Geometry check sheet. Reference: the model listing, model coordinates, mm. A direction names the side the tool comes from. Round coordinates to 2 decimals unless told otherwise and drop trailing zeros. Loops run counter-clockwise (first coordinate to the right, second up) from the corner with the lowest first, then second, coordinate; pieces in that order, holes last. Notation, with made-up numbers: (50.25, 52) -> (75.25, 52) arc R21 cw to (75.25, 79) -> close; hole circle Ø3 at (-32.5, -30). An arc over 180 degrees is marked (long way). Use a Markdown table: item, result. Add a question column.
Q1. Sectioned sample at A-A, the plane z = -48.5. Enter the section's corners in (x, y).
Q2. Release check for a two-part mould opening along Z. For faces 4 (the face through (16.25, 1.52, -310.3)), 5 (the face through (203.75, 1.52, -9.7)), 6 (the face through (41.01, 1.52, -283.15)) record: released by +Z, released by -Z, zero draft, split by the parting line, or undercut.
Q3. Set-up check for faces 1 (the face through (9.67, 1.52, -18.96)), 2 (the face through (47.85, 1.52, -207.99)), 3 (the face through (16.065, 1.521, -9.482)): record each of +Z, -Z, +X, -X, +Y, -Y from which the full face is reachable in a straight line by a thin tool's end or side.
Q4. Material ranges on L1, parallel to X at y = 2.05, z = -119.5; L2, parallel to X at y = 2.35, z = -44; L3, parallel to X at y = 1.6, z = -104.5, recorded low to high.
Q5. Sectioned sample at C-C, the plane y = 2.05. Give the number of separate pieces and of enclosed holes in the cut face, then the cut area to 3 significant figures.
Q6. Sectioned sample at B-B, the plane x = 144.5. Enter the section's corners in (y, z), then the cut area to 3 significant figures.
Q7. Gauge pin test, flat ends, axial feed: P1, Ø1.5, axis at y = 2, z = -136.5, coming from the -X side; P2, Ø1.5, axis at x = 23, y = 1.5, coming from the -Z side; P3, Ø0.9, axis at y = 2, z = -189, coming from the +X side. Record the tip position at first contact, or that the pin passes through.
```python
from build123d import *

# Parameters (mm, degrees)
CROQUIS1_W              = 220
CROQUIS1_H              = 320
CROQUIS1_R              = 1.7
CROQUIS1_R_2            = 1.6
SALIENTE_EXTRUIR1_DEPTH = 3
CROQUIS2_OUTSIDE_W      = 299.668
CROQUIS2_OUTSIDE_H      = 399.668
CORTAR_EXTRUIR1_DEPTH   = 3
REDONDEO1_R             = 5
CROQUIS3_W              = 20
CROQUIS3_H              = 45
CORTAR_EXTRUIR2_DEPTH   = 3
CROQUIS4_W              = 15
CROQUIS4_H              = 60
CORTAR_EXTRUIR3_DEPTH   = 3
REDONDEO2_R             = 5


with BuildPart() as part:
    # Croquis1 → Saliente-Extruir1 (new body)
    with BuildSketch(Plane(origin=(0, 0, 0), x_dir=(1, 0, 0), z_dir=(0, 1, 0))):
        with Locations((110, 160)):
            Rectangle(CROQUIS1_W, CROQUIS1_H)
        with Locations(Location((185, 167.5, 0), (0, 0, 270))):
            Circle(CROQUIS1_R, mode=Mode.SUBTRACT)
        with Locations(Location((205, 167.5, 0), (0, 0, 270))):
            Circle(CROQUIS1_R, mode=Mode.SUBTRACT)
        with Locations(Location((185, 152.5, 0), (0, 0, 90))):
            Circle(CROQUIS1_R, mode=Mode.SUBTRACT)
        with Locations(Location((205, 152.5, 0), (0, 0, 90))):
            Circle(CROQUIS1_R, mode=Mode.SUBTRACT)
        with Locations(Location((35, 215.5, 0), (0, 0, 270))):
            Circle(CROQUIS1_R, mode=Mode.SUBTRACT)
        with Locations(Location((35, 200.5, 0), (0, 0, 270))):
            Circle(CROQUIS1_R, mode=Mode.SUBTRACT)
        with Locations(Location((35, 119.5, 0), (0, 0, 90))):
            Circle(CROQUIS1_R, mode=Mode.SUBTRACT)
        with Locations(Location((35, 104.5, 0), (0, 0, 90))):
            Circle(CROQUIS1_R, mode=Mode.SUBTRACT)
        with Locations(Location((5.5, 314.5, 0), (0, 0, 270))):
            Circle(CROQUIS1_R_2, mode=Mode.SUBTRACT)
        with Locations(Location((214.5, 314.5, 0), (0, 0, 90))):
            Circle(CROQUIS1_R_2, mode=Mode.SUBTRACT)
        with Locations(Location((214.5, 5.5, 0), (0, 0, 270))):
            Circle(CROQUIS1_R_2, mode=Mode.SUBTRACT)
        with Locations(Location((5.5, 5.5, 0), (0, 0, 90))):
            Circle(CROQUIS1_R_2, mode=Mode.SUBTRACT)
        with Locations(Location((15, 200.5, 0), (0, 0, 90))):
            Circle(CROQUIS1_R, mode=Mode.SUBTRACT)
        with Locations(Location((15, 215.5, 0), (0, 0, 90))):
            Circle(CROQUIS1_R, mode=Mode.SUBTRACT)
        with Locations(Location((15, 104.5, 0), (0, 0, 270))):
            Circle(CROQUIS1_R, mode=Mode.SUBTRACT)
        with Locations(Location((15, 119.5, 0), (0, 0, 270))):
            Circle(CROQUIS1_R, mode=Mode.SUBTRACT)
        with Locations(Location((110, 180, 0), (0, 0, 270))):
            Circle(CROQUIS1_R_2, mode=Mode.SUBTRACT)
        with Locations(Location((110, 140, 0), (0, 0, 90))):
            Circle(CROQUIS1_R_2, mode=Mode.SUBTRACT)
        with Locations(Location((5.5, 160, 0), (0, 0, 270))):
            Circle(CROQUIS1_R_2, mode=Mode.SUBTRACT)
        with Locations(Location((214.5, 160, 0), (0, 0, 90))):
            Circle(CROQUIS1_R_2, mode=Mode.SUBTRACT)
    extrude(amount=SALIENTE_EXTRUIR1_DEPTH)

    # Croquis2 outside → Cortar-Extruir1 (cut)
    # profile 1 of 9: a face of its own
    with BuildSketch(Plane(origin=(0, 3, 0), x_dir=(1, 0, 0), z_dir=(0, 1, 0))):
        with Locations((110, 160)):
            Rectangle(CROQUIS2_OUTSIDE_W, CROQUIS2_OUTSIDE_H)
        with BuildLine():
            Line((9, 148.77502784), (9, 94.5))
            Line((9, 94.5), (19, 94.5))
            Line((19, 94.5), (19, 30))
            Line((19, 30), (1.298802547, 9.049639413))
            ThreePointArc((1.298802547, 9.049639413), (1.950360587, 1.298802547), (9.701197453, 1.950360587))
            Line((9.701197453, 1.950360587), (24.106631311, 19))
            Line((24.106631311, 19), (195.893368689, 19))
            Line((195.893368689, 19), (210.298802547, 1.950360587))
            ThreePointArc((210.298802547, 1.950360587), (218.049639413, 1.298802547), (218.701197453, 9.049639413))
            Line((218.701197453, 9.049639413), (201, 30))
            Line((201, 30), (201, 94.5))
            Line((201, 94.5), (211, 94.5))
            Line((211, 94.5), (211, 148.77502784))
            ThreePointArc((211, 148.77502784), (212.318863014, 152.528287293), (215.695652174, 154.631535054))
            ThreePointArc((215.695652174, 154.631535054), (220, 160), (215.695652174, 165.368464946))
            ThreePointArc((215.695652174, 165.368464946), (212.318863014, 167.471712707), (211, 171.22497216))
            Line((211, 171.22497216), (211, 225.5))
            Line((211, 225.5), (201, 225.5))
            Line((201, 225.5), (201, 290))
            Line((201, 290), (218.701197453, 310.950360587))
            ThreePointArc((218.701197453, 310.950360587), (218.049639413, 318.701197453), (210.298802547, 318.049639413))
            Line((210.298802547, 318.049639413), (195.893368689, 301))
            Line((195.893368689, 301), (24.106631311, 301))
            Line((24.106631311, 301), (9.701197453, 318.049639413))
            ThreePointArc((9.701197453, 318.049639413), (1.950360587, 318.701197453), (1.298802547, 310.950360587))
            Line((1.298802547, 310.950360587), (19, 290))
            Line((19, 290), (19, 225.5))
            Line((19, 225.5), (9, 225.5))
            Line((9, 225.5), (9, 171.22497216))
            ThreePointArc((9, 171.22497216), (7.681136986, 167.471712707), (4.304347826, 165.368464946))
            ThreePointArc((4.304347826, 165.368464946), (0, 160), (4.304347826, 154.631535054))
            ThreePointArc((4.304347826, 154.631535054), (7.681136986, 152.528287293), (9, 148.77502784))
        make_face(mode=Mode.SUBTRACT)
    # profile 2 of 9: a face of its own
    with BuildSketch(Plane(origin=(0, 3, 0), x_dir=(1, 0, 0), z_dir=(0, 1, 0))):
        with BuildLine():
            Line((182, 276), (182, 236))
            ThreePointArc((182, 236), (179.071067812, 228.928932188), (172, 226))
            Line((172, 226), (118, 226))
            ThreePointArc((118, 226), (116.585786438, 226.585786438), (116, 228))
            Line((116, 228), (116, 284))
            ThreePointArc((116, 284), (116.585786438, 285.414213562), (118, 286))
            Line((118, 286), (172, 286))
            ThreePointArc((172, 286), (179.071067812, 283.071067812), (182, 276))
        make_face()
    # profile 3 of 9: a face of its own
    with BuildSketch(Plane(origin=(0, 3, 0), x_dir=(1, 0, 0), z_dir=(0, 1, 0))):
        with BuildLine():
            Line((102, 286), (48, 286))
            ThreePointArc((48, 286), (40.928932188, 283.071067812), (38, 276))
            Line((38, 276), (38, 236))
            ThreePointArc((38, 236), (40.928932188, 228.928932188), (48, 226))
            Line((48, 226), (102, 226))
            ThreePointArc((102, 226), (103.414213562, 226.585786438), (104, 228))
            Line((104, 228), (104, 284))
            ThreePointArc((104, 284), (103.414213562, 285.414213562), (102, 286))
        make_face()
    # profile 4 of 9: a face of its own
    with BuildSketch(Plane(origin=(0, 3, 0), x_dir=(1, 0, 0), z_dir=(0, 1, 0))):
        with BuildLine():
            Line((102, 94), (48, 94))
            ThreePointArc((48, 94), (40.928932188, 91.071067812), (38, 84))
            Line((38, 84), (38, 44))
            ThreePointArc((38, 44), (40.928932188, 36.928932188), (48, 34))
            Line((48, 34), (102, 34))
            ThreePointArc((102, 34), (103.414213562, 34.585786438), (104, 36))
            Line((104, 36), (104, 92))
            ThreePointArc((104, 92), (103.414213562, 93.414213562), (102, 94))
        make_face()
    # profile 5 of 9: a face of its own
    with BuildSketch(Plane(origin=(0, 3, 0), x_dir=(1, 0, 0), z_dir=(0, 1, 0))):
        with BuildLine():
            Line((116, 36), (116, 92))
            ThreePointArc((116, 92), (116.585786438, 93.414213562), (118, 94))
            Line((118, 94), (172, 94))
            ThreePointArc((172, 94), (179.071067812, 91.071067812), (182, 84))
            Line((182, 84), (182, 44))
            ThreePointArc((182, 44), (179.071067812, 36.928932188), (172, 34))
            Line((172, 34), (118, 34))
            ThreePointArc((118, 34), (116.585786438, 34.585786438), (116, 36))
        make_face()
    # profile 6 of 9: a face of its own
    with BuildSketch(Plane(origin=(0, 3, 0), x_dir=(1, 0, 0), z_dir=(0, 1, 0))):
        with BuildLine():
            Line((45, 152), (45, 119))
            ThreePointArc((45, 119), (47.928932188, 111.928932188), (55, 109))
            Line((55, 109), (85, 109))
            ThreePointArc((85, 109), (92.071067812, 111.928932188), (95, 119))
            Line((95, 119), (95, 152))
            ThreePointArc((95, 152), (94.414213562, 153.414213562), (93, 154))
            Line((93, 154), (47, 154))
            ThreePointArc((47, 154), (45.585786438, 153.414213562), (45, 152))
        make_face()
    # profile 7 of 9: a face of its own
    with BuildSketch(Plane(origin=(0, 3, 0), x_dir=(1, 0, 0), z_dir=(0, 1, 0))):
        with BuildLine():
            Line((93, 166), (47, 166))
            ThreePointArc((47, 166), (45.585786438, 166.585786438), (45, 168))
            Line((45, 168), (45, 201))
            ThreePointArc((45, 201), (47.928932188, 208.071067812), (55, 211))
            Line((55, 211), (85, 211))
            ThreePointArc((85, 211), (92.071067812, 208.071067812), (95, 201))
            Line((95, 201), (95, 168))
            ThreePointArc((95, 168), (94.414213562, 166.585786438), (93, 166))
        make_face()
    # profile 8 of 9: a face of its own
    with BuildSketch(Plane(origin=(0, 3, 0), x_dir=(1, 0, 0), z_dir=(0, 1, 0))):
        with BuildLine():
            Line((135, 109), (165, 109))
            ThreePointArc((165, 109), (172.071067812, 111.928932188), (175, 119))
            Line((175, 119), (175, 152))
            ThreePointArc((175, 152), (174.414213562, 153.414213562), (173, 154))
            Line((173, 154), (127, 154))
            ThreePointArc((127, 154), (125.585786438, 153.414213562), (125, 152))
            Line((125, 152), (125, 119))
            ThreePointArc((125, 119), (127.928932188, 111.928932188), (135, 109))
        make_face()
    # profile 9 of 9: a face of its own
    with BuildSketch(Plane(origin=(0, 3, 0), x_dir=(1, 0, 0), z_dir=(0, 1, 0))):
        with BuildLine():
            Line((127, 166), (173, 166))
            ThreePointArc((173, 166), (174.414213562, 166.585786438), (175, 168))
            Line((175, 168), (175, 201))
            ThreePointArc((175, 201), (172.071067812, 208.071067812), (165, 211))
            Line((165, 211), (135, 211))
            ThreePointArc((135, 211), (127.928932188, 208.071067812), (125, 201))
            Line((125, 201), (125, 168))
            ThreePointArc((125, 168), (125.585786438, 166.585786438), (127, 166))
        make_face()
    extrude(amount=-CORTAR_EXTRUIR1_DEPTH, mode=Mode.SUBTRACT)

    # Redondeo1
    redondeo1_edges = [part.edges().sort_by_distance(p)[0] for p in [
        (9, 1.5, -225.5),
        (9, 1.5, -94.5),
        (24.106631311, 1.5, -301),
        (195.893368689, 1.5, -301),
        (201, 1.5, -290),
        (201, 1.5, -30),
        (195.893368689, 1.5, -19),
        (24.106631311, 1.5, -19),
        (19, 1.5, -30),
        (19, 1.5, -94.5),
        (19, 1.5, -290),
        (19, 1.5, -225.5),
    ]]
    fillet(redondeo1_edges, radius=REDONDEO1_R - 0.0001)  # a hair under: the kernel refuses the full size

    # Croquis3 → Cortar-Extruir2 (cut)
    with BuildSketch(Plane(origin=(0, 3, 0), x_dir=(1, 0, 0), z_dir=(0, 1, 0))):
        with Locations((201, 203)):
            Rectangle(CROQUIS3_W, CROQUIS3_H)
        with Locations((201, 117)):
            Rectangle(CROQUIS3_W, CROQUIS3_H)
    extrude(amount=-CORTAR_EXTRUIR2_DEPTH, mode=Mode.SUBTRACT)

    # Croquis4 → Cortar-Extruir3 (cut)
    with BuildSketch(Plane(origin=(0, 3, 0), x_dir=(1, 0, 0), z_dir=(0, 1, 0))):
        with Locations((24.5, 160)):
            Rectangle(CROQUIS4_W, CROQUIS4_H)
    extrude(amount=-CORTAR_EXTRUIR3_DEPTH, mode=Mode.SUBTRACT)

    # Redondeo2
    redondeo2_edges = [part.edges().sort_by_distance(p)[0] for p in [
        (201, 1.5, -94.5),
        (191, 1.5, -94.5),
        (191, 1.5, -139.5),
        (211, 1.5, -139.5),
        (211, 1.5, -180.5),
        (191, 1.5, -180.5),
        (191, 1.5, -225.5),
        (201, 1.5, -225.5),
        (32, 1.5, -190),
        (17, 1.5, -190),
        (17, 1.5, -130),
        (32, 1.5, -130),
    ]]
    fillet(redondeo2_edges, radius=REDONDEO2_R - 0.0001)  # a hair under: the kernel refuses the full size


solid = part.part
```
Values:
| question | item | result |
|---|---|---|
| 1 | outline | (19, 0) -> (38, 0) -> (38, 3) -> (19, 3) -> close; (104, 0) -> (116, 0) -> (116, 3) -> (104, 3) -> close; (182, 0) -> (201, 0) -> (201, 3) -> (182, 3) -> close |
| 2 | face 4 | released by -Z |
| 2 | face 5 | released by +Z |
| 2 | face 6 | undercut |
| 3 | face 1 | -X, +Y, -Y |
| 3 | face 2 | +Y, -Y |
| 3 | face 3 | +Z, +Y, -Y |
| 4 | L1 | 9 to 13.3, 16.7 to 33.3, 36.7 to 45, 95 to 125, 175 to 191 |
| 4 | L2 | 19 to 38, 104 to 116, 182 to 201 |
| 4 | L3 | 9 to 13.3, 16.7 to 33.3, 36.7 to 191 |
| 5 | separate pieces | 1 |
| 5 | enclosed holes | 29 |
| 5 | area | 28,000 mm^2 |
| 6 | outline | (0, -301) -> (3, -301) -> (3, -286) -> (0, -286) -> close; (0, -226) -> (3, -226) -> (3, -211) -> (0, -211) -> close; (0, -166) -> (3, -166) -> (3, -154) -> (0, -154) -> close; (0, -109) -> (3, -109) -> (3, -94) -> (0, -94) -> close; (0, -34) -> (3, -34) -> (3, -19) -> (0, -19) -> close |
| 6 | area | 216 mm^2 |
| 7 | P1 | x = 9 |
| 7 | P2 | z = -303.2 |
| 7 | P3 | x = 191 |
